```python
from build123d import *

# Parameters (mm, degrees)
SKETCH_1_W               = 33
SKETCH_1_H               = 37
EXTRUDE_1_DEPTH          = 38
CUT_EXTRUDE_1_DEPTH      = 54.930510845
CUT_EXTRUDE_2_DEPTH      = 54.930510845
CUT_EXTRUDE_2_DEPTH_BACK = 54.930510845
SKETCH_3_W               = 46
SKETCH_3_H               = 9
SKETCH_4_W               = 17
SKETCH_4_H               = 37
CUT_EXTRUDE_3_DEPTH      = 6
SKETCH_5_R               = 6
CUT_EXTRUDE_4_DEPTH      = 50.884867445


with BuildPart() as part:
    # 草图1 → 凸台-拉伸1 (new body)
    with BuildSketch(Plane(origin=(0, 0, 0), x_dir=(1, 0, 0), z_dir=(0, 1, 0))):
        Polygon((-33.5, -10), (-33.5, 10), (-16.5, 18.5), (-16.5, -18.5), align=None)
        Rectangle(SKETCH_1_W, SKETCH_1_H)
        Polygon((33.5, -10), (16.5, -18.5), (16.5, 18.5), (33.5, 10), align=None)
    extrude(amount=EXTRUDE_1_DEPTH)

    # 草图2 → 切除-拉伸1 (cut, symmetric)
    with BuildSketch(Plane.XY):
        Polygon((-80.545432509, 152.17109707), (16.5, 38), (33.5, 18), (130.545432509, -96.17109707), (358.887626649, 97.919767949), (147.79676163, 346.261962088), align=None)
    cut_extrude_1 = extrude(amount=CUT_EXTRUDE_1_DEPTH, both=True, mode=Mode.SUBTRACT)

    # 镜向1: 切除-拉伸1 across plane
    add(cut_extrude_1.mirror(Plane(origin=(0, 0, 0), x_dir=(0, 0, 1), z_dir=(1, 0, 0))), mode=Mode.SUBTRACT)

    # 草图3 → 切除-拉伸2 (cut, two sides: drawn at the far end of the back side and taken through both)
    with BuildSketch(Plane.XY.offset(-CUT_EXTRUDE_2_DEPTH_BACK)):
        with Locations((0, 4.5)):
            Rectangle(SKETCH_3_W, SKETCH_3_H)
    extrude(amount=CUT_EXTRUDE_2_DEPTH + CUT_EXTRUDE_2_DEPTH_BACK, mode=Mode.SUBTRACT)

    # 草图4 → 切除-拉伸3 (cut)
    with BuildSketch(Plane(origin=(0, 38, 0), x_dir=(1, 0, 0), z_dir=(0, 1, 0))):
        Rectangle(SKETCH_4_W, SKETCH_4_H)
    extrude(amount=-CUT_EXTRUDE_3_DEPTH, mode=Mode.SUBTRACT)

    # 草图5 → 切除-拉伸4 (cut, through all)
    with BuildSketch(Plane(origin=(0, 32, 0), x_dir=(1, 0, 0), z_dir=(0, 1, 0))):
        with Locations(Location((0, 0, 0), (0, 0, 270))):
            Circle(SKETCH_5_R)
    extrude(amount=-CUT_EXTRUDE_4_DEPTH, mode=Mode.SUBTRACT)


solid = part.part
```
Build history of the part. All positions in model axes, mm. A direction names the side the tool comes from. Coordinates: 2 decimals unless noted, no trailing zeros. Order: outer loops, then holes, each group sorted by start corner. A loop starts at its lowest first (then second) coordinate and runs counter-clockwise, first axis right, second up. Notation, with made-up numbers: (40.5, -16.75) -> (72.5, -16.75) arc R15 ccw to (72.5, -0.75) -> close; hole circle Ø8 at (81.25, -29). An arc over 180 degrees is marked (long way). Answer in a Markdown table with one row per item. Add a question column.
Q1. Band-saw the part on C-C, the plane y = 11.5. List the corners of the cut face in (x, z).
Q2. Band-saw the part on B-B, the plane x = 0. List the corners of the cut face in (y, z), then the cut area to 3 significant figures.
Q3. Which spindle directions (+Z, -Z, +X, -X, +Y, -Y) get a long thin tool onto all of the face, cutting with end or side? Do faces 1 (the face through (24.9, 14.5, -14.3)), 2 (the face through (-5, 9, 4)), 3 (the face through (-8.5, 35, 0)). Say none if no direction does.
Q4. Drop flat-ended pins along their axis: pin 1 (1.8 mm diameter, centred on y = 35.5, z = 8.5, fed in from -X); pin 2 (5 mm diameter, centred on x = 1.5, z = 2, fed in from +Y); pin 3 (18.5 mm diameter, centred on x = -1.5, z = 2, fed in from -Y); pin 4 (2 mm diameter, centred on y = 28.5, z = 5, fed in from -X) (3 decimals). Give the stop position or say it passes through.
Q5. Band-saw the part on A-A, the plane y = 3. List the corners of the cut face in (x, z), then the cut area to 3 significant figures.
Q6. Wall check: line 1 along X through (y, z) = (5, 4); line 2 along Y through (x, z) = (-6, 6); line 3 along X through (y, z) = (18, 0). Give the ranges that are in metal, low to high. Write a range as [from, to].
Q7. Mould opens along X. For faces 4 (the face through (-23, 4, 0)), 5 (the face through (13, 38, 0)), 6 (the face through (-22.992, 30.362, 0.259)) say: +X half, -X half, draft (parallel to the pull), parting line (faces both ways), or undercut.
Q8. Band-saw the part on D-D, the plane z = 0. List the corners of the cut face in (x, y), then the cut area to 3 significant figures.
Answers follow:
| question | item | result |
|---|---|---|
| 1 | outline | (-33.5, -10) -> (-16.5, -18.5) -> (16.5, -18.5) -> (33.5, -10) -> (33.5, 10) -> (16.5, 18.5) -> (-16.5, 18.5) -> (-33.5, 10) -> close; hole circle Ø12 at (0, 0) |
| 2 | outline | (9, -18.5) -> (32, -18.5) -> (32, -6) -> (9, -6) -> close; (9, 6) -> (32, 6) -> (32, 18.5) -> (9, 18.5) -> close |
| 2 | area | 575 mm^2 |
| 3 | face 1 | -Z, +X, +Y, -Y |
| 3 | face 2 | +Z, -Z, -Y |
| 3 | face 3 | +Z, -Z, +Y |
| 4 | pin 1 | x = -19.39 |
| 4 | pin 2 | through |
| 4 | pin 3 | y = 9 |
| 4 | pin 4 | x = -25.425 |
| 5 | outline | (-33.5, -10) -> (-23, -15.25) -> (-23, 15.25) -> (-33.5, 10) -> close; (23, -15.25) -> (33.5, -10) -> (33.5, 10) -> (23, 15.25) -> close |
| 5 | area | 530 mm^2 |
| 6 | line 1 | [-33.5, -23], [23, 33.5] |
| 6 | line 2 | [9, 32] |
| 6 | line 3 | [-33.5, -6], [6, 33.5] |
| 7 | face 4 | undercut |
| 7 | face 5 | draft |
| 7 | face 6 | -X half |
| 8 | outline | (-33.5, 0) -> (-23, 0) -> (-23, 9) -> (-6, 9) -> (-6, 32) -> (-8.5, 32) -> (-8.5, 38) -> (-16.5, 38) -> (-33.5, 18) -> close; (6, 9) -> (23, 9) -> (23, 0) -> (33.5, 0) -> (33.5, 18) -> (16.5, 38) -> (8.5, 38) -> (8.5, 32) -> (6, 32) -> close |
| 8 | area | 1,410 mm^2 |
